CAD build for the part. Positions are in the model's coordinates, mm. Face numbers are marked on the shaded views. A direction names the side the tool comes from. Round coordinates to 2 decimals unless told otherwise and drop trailing zeros. Loops run counter-clockwise (first coordinate to the right, second up) from the corner with the lowest first, then second, coordinate; pieces in that order, holes last.
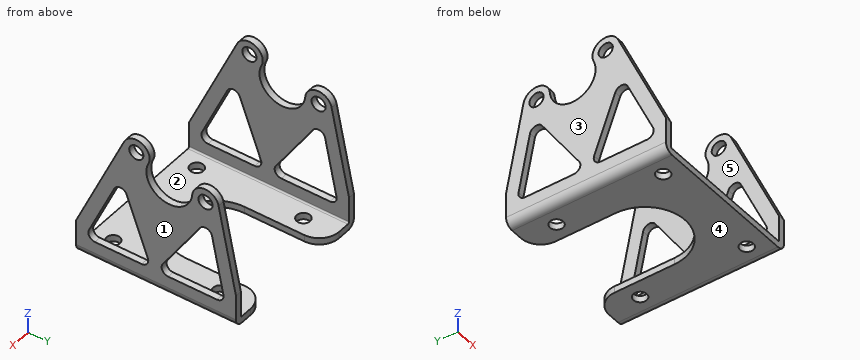
```python
from build123d import *

# Parameters (mm, degrees)
SKETCH4_R                      = 3.175
BASE_FLANGE1_DEPTH             = 3.175
EDGE_FLANGE1_STRIP_W           = 14.1732
EDGE_FLANGE1_STRIP_H           = 3.175
EDGE_FLANGE1_STRIP_CUT_DEPTH   = 76.2
EDGE_FLANGE1_STRIP_2_W         = 14.1732
EDGE_FLANGE1_STRIP_2_H         = 3.175
EDGE_FLANGE1_STRIP_CUT_2_DEPTH = 76.2
EDGE_FLANGE1_DEPTH             = 76.2
EDGE_FLANGE1_BEND_DEPTH        = 76.2
CUT_EXTRUDE2_DEPTH             = 113.499830191
CUT_EXTRUDE3_REACH             = 110.728
SKETCH21_R                     = 3.3782


# Sheet-metal steps are written as plain solids
with BuildPart() as part:
    # Sketch4 → Base-Flange1 (new body)
    with BuildSketch(Plane.XY):
        with BuildLine():
            Line((38.470301513, 37.249760359), (28.945301513, 37.249760359))
            ThreePointArc((28.945301513, 37.249760359), (22.210109423, 34.45995245), (19.420301513, 27.724760359))
            Line((19.420301513, 27.724760359), (19.420301513, -0.850239641))
            ThreePointArc((19.420301513, -0.850239641), (0.370301513, -19.900239641), (-18.679698487, -0.850239641))
            Line((-18.679698487, -0.850239641), (-18.679698487, 27.724760359))
            ThreePointArc((-18.679698487, 27.724760359), (-21.469506396, 34.45995245), (-28.204698487, 37.249760359))
            Line((-28.204698487, 37.249760359), (-37.729698487, 37.249760359))
            Line((-37.729698487, 37.249760359), (-37.729698487, -38.950239641))
            Line((-37.729698487, -38.950239641), (38.470301513, -38.950239641))
            Line((38.470301513, -38.950239641), (38.470301513, 37.249760359))
        make_face()
        with Locations((-26.617198487, -29.425239641)):
            Circle(SKETCH4_R, mode=Mode.SUBTRACT)
        with Locations((27.357801513, -29.425239641)):
            Circle(SKETCH4_R, mode=Mode.SUBTRACT)
        with Locations((27.357801513, 21.374760359)):
            Circle(SKETCH4_R, mode=Mode.SUBTRACT)
        with Locations((-26.617198487, 21.374760359)):
            Circle(SKETCH4_R, mode=Mode.SUBTRACT)
    extrude(amount=-BASE_FLANGE1_DEPTH)

    # Edge-Flange1 strip (across the edge) → Edge-Flange1 strip cut (cut)
    with BuildSketch(Plane(origin=(38.470301513, -38.950239641, 0), x_dir=(-1, 0, 0), z_dir=(0, 1, 0))):
        with Locations((-3.175, -1.5875)):
            Rectangle(EDGE_FLANGE1_STRIP_W, EDGE_FLANGE1_STRIP_H)
    extrude(amount=EDGE_FLANGE1_STRIP_CUT_DEPTH, mode=Mode.SUBTRACT)

    # Edge-Flange1 strip 2 (across the edge) → Edge-Flange1 strip cut 2 (cut)
    with BuildSketch(Plane(origin=(-37.729698487, 37.249760359, 0), x_dir=(1, 0, 0), z_dir=(0, -1, 0))):
        with Locations((-3.175, -1.5875)):
            Rectangle(EDGE_FLANGE1_STRIP_2_W, EDGE_FLANGE1_STRIP_2_H)
    extrude(amount=EDGE_FLANGE1_STRIP_CUT_2_DEPTH, mode=Mode.SUBTRACT)

    # Edge-Flange1 section (across the edge) → Edge-Flange1 (add)
    with BuildSketch(Plane(origin=(38.470301513, -38.950239641, 0), x_dir=(-1, 0, 0), z_dir=(0, 1, 0))):
        with BuildLine():
            Line((0, 0.7366), (0, 73.025))
            Line((0, 73.025), (3.175, 73.025))
            Line((3.175, 73.025), (3.175, 0.7366))
            ThreePointArc((3.175, 0.7366), (3.390745145, 0.215745145), (3.9116, 0))
            Line((3.9116, 0), (3.9116, -3.175))
            ThreePointArc((3.9116, -3.175), (1.145681115, -2.029318885), (0, 0.7366))
        make_face()
    extrude(amount=EDGE_FLANGE1_DEPTH)

    # Edge-Flange1 section 2 (across the edge) → Edge-Flange1 bend (add)
    with BuildSketch(Plane(origin=(-37.729698487, 37.249760359, 0), x_dir=(1, 0, 0), z_dir=(0, -1, 0))):
        with BuildLine():
            Line((0, 0.7366), (0, 73.025))
            Line((0, 73.025), (3.175, 73.025))
            Line((3.175, 73.025), (3.175, 0.7366))
            ThreePointArc((3.175, 0.7366), (3.390745145, 0.215745145), (3.9116, 0))
            Line((3.9116, 0), (3.9116, -3.175))
            ThreePointArc((3.9116, -3.175), (1.145681115, -2.029318885), (0, 0.7366))
        make_face()
    extrude(amount=EDGE_FLANGE1_BEND_DEPTH)

    # Sketch18 → Cut-Extrude2 (cut, through all)
    with BuildSketch(Plane(origin=(38.470301513, 0, 0), x_dir=(0, 0, -1), z_dir=(1, 0, 0))):
        with BuildLine():
            Line((-12.7, 37.249760359), (-53.545242344, 28.944361059))
            ThreePointArc((-53.545242344, 28.944361059), (-58.617648241, 22.326829154), (-52.763048756, 16.390104891))
            ThreePointArc((-52.763048756, 16.390104891), (-43.013397441, 2.790344649), (-58.09955595, -4.449613972))
            ThreePointArc((-58.09955595, -4.449613972), (-66.503585183, -7.614624659), (-63.338574497, -16.018653892))
            Line((-63.338574497, -16.018653892), (-12.7, -38.950239641))
            Line((-12.7, -38.950239641), (-73.025, -38.950239641))
            Line((-73.025, -38.950239641), (-73.025, 37.249760359))
            Line((-73.025, 37.249760359), (-12.7, 37.249760359))
        make_face()
    extrude(amount=-CUT_EXTRUDE2_DEPTH, mode=Mode.SUBTRACT)

    # Cut-Extrude3: up to this face of the body (flat: up to its plane)
    cut_extrude3_end = Plane(part.part.faces().sort_by_distance((-37.729698487, 0.375360162, 25.894827333))[0])
    # Sketch21 → Cut-Extrude3 (cut, up to the picked face)
    with BuildSketch(Plane(origin=(38.470301513, 0, 0), x_dir=(0, 0, -1), z_dir=(1, 0, 0)), mode=Mode.PRIVATE) as cut_extrude3_sk1:
        with Locations((-60.719065223, -10.234133932)):
            Circle(SKETCH21_R)
    cut_extrude3_tool1 = split(extrude(cut_extrude3_sk1.sketch, amount=-CUT_EXTRUDE3_REACH, mode=Mode.PRIVATE), bisect_by=cut_extrude3_end, keep=Keep.BOTH, mode=Mode.PRIVATE)
    # Sketch21 → Cut-Extrude3 (cut, up to the picked face)
    with BuildSketch(Plane(origin=(38.470301513, 0, 0), x_dir=(0, 0, -1), z_dir=(1, 0, 0)), mode=Mode.PRIVATE) as cut_extrude3_sk2:
        with Locations((-52.279937568, 22.721700549)):
            Circle(SKETCH21_R)
    cut_extrude3_tool2 = split(extrude(cut_extrude3_sk2.sketch, amount=-CUT_EXTRUDE3_REACH, mode=Mode.PRIVATE), bisect_by=cut_extrude3_end, keep=Keep.BOTH, mode=Mode.PRIVATE)
    # Sketch21 → Cut-Extrude3 (cut, up to the picked face)
    with BuildSketch(Plane(origin=(38.470301513, 0, 0), x_dir=(0, 0, -1), z_dir=(1, 0, 0)), mode=Mode.PRIVATE) as cut_extrude3_sk3:
        with BuildLine():
            Line((-10.64400026, -4.738220863), (-37.435582613, -14.828100623))
            ThreePointArc((-37.435582613, -14.828100623), (-39.489903551, -17.696138128), (-37.62633699, -20.691633633))
            Line((-37.62633699, -20.691633633), (-10.834754637, -32.824152651))
            ThreePointArc((-10.834754637, -32.824152651), (-7.804221974, -32.600140782), (-6.35, -29.931892671))
            Line((-6.35, -29.931892671), (-6.35, -7.709493893))
            ThreePointArc((-6.35, -7.709493893), (-7.718373423, -5.09860795), (-10.64400026, -4.738220863))
        make_face()
    cut_extrude3_tool3 = split(extrude(cut_extrude3_sk3.sketch, amount=-CUT_EXTRUDE3_REACH, mode=Mode.PRIVATE), bisect_by=cut_extrude3_end, keep=Keep.BOTH, mode=Mode.PRIVATE)
    # Sketch21 → Cut-Extrude3 (cut, up to the picked face)
    with BuildSketch(Plane(origin=(38.470301513, 0, 0), x_dir=(0, 0, -1), z_dir=(1, 0, 0)), mode=Mode.PRIVATE) as cut_extrude3_sk4:
        with BuildLine():
            Line((-38.069272281, 20.080292762), (-11.277689928, 2.343110591))
            ThreePointArc((-11.277689928, 2.343110591), (-8.022363238, 2.193595711), (-6.35, 4.990506107))
            Line((-6.35, 4.990506107), (-6.35, 28.175441224))
            ThreePointArc((-6.35, 28.175441224), (-7.516025925, 30.634027844), (-10.157652388, 31.286771479))
            Line((-10.157652388, 31.286771479), (-36.949234742, 25.839018533))
            ThreePointArc((-36.949234742, 25.839018533), (-39.433182282, 23.333848227), (-38.069272281, 20.080292762))
        make_face()
    cut_extrude3_tool4 = split(extrude(cut_extrude3_sk4.sketch, amount=-CUT_EXTRUDE3_REACH, mode=Mode.PRIVATE), bisect_by=cut_extrude3_end, keep=Keep.BOTH, mode=Mode.PRIVATE)
    add(cut_extrude3_tool1.solids().sort_by(Axis((38.470302, -10.234134, 60.719065), (-1, 0, 0)))[0], mode=Mode.SUBTRACT)
    add(cut_extrude3_tool2.solids().sort_by(Axis((38.470302, 22.721701, 52.279938), (-1, 0, 0)))[0], mode=Mode.SUBTRACT)
    add(cut_extrude3_tool3.solids().sort_by(Axis((38.470302, -18.49522, 18.845957), (-1, 0, 0)))[0], mode=Mode.SUBTRACT)
    add(cut_extrude3_tool4.solids().sort_by(Axis((38.470302, 18.532132, 18.821153), (-1, 0, 0)))[0], mode=Mode.SUBTRACT)


solid = part.part
```
Item 1: Cut at B-B, the plane z = 21. Give the cut face in (x, y).
Answers follow:
outline: (-37.73, -35.19) - (-34.55, -35.19) - (-34.55, -28.22) - (-37.73, -28.22) - close; (-37.73, -8.64) - (-34.55, -8.64) - (-34.55, 8.78) - (-37.73, 8.78) - close; (-37.73, 29.08) - (-34.55, 29.08) - (-34.55, 35.56) - (-37.73, 35.56) - close; (35.3, -35.19) - (38.47, -35.19) - (38.47, -28.22) - (35.3, -28.22) - close; (35.3, -8.64) - (38.47, -8.64) - (38.47, 8.78) - (35.3, 8.78) - close; (35.3, 29.08) - (38.47, 29.08) - (38.47, 35.56) - (35.3, 35.56) - close
Item 2: 3-axis set-ups, long thin cutter, end or side, ignore diameter. For the marked faces 1 and 2: which of +Z, -Z, +X, -X, +Y, -Y reach the whole face in a straight line?
Answers follow:
face 1: +Z, -Z, +X, +Y, -Y
face 2: +Z, +Y, -Y
Item 3: Two-plate mould, pull along X, no slides. Class the marked faces 3, 4 and 5: released by +X, released by -X, zero draft, split by the parting line, or undercut.
Answers follow:
face 3: released by -X
face 4: zero draft
face 5: undercut
Item 4: Cut at D-D, the plane x = 27.5. Give the cut face in (y, z) (3 decimals), plus the area to 3 significant figures.
Answers follow:
outline: (-38.95, -3.175) - (-32.597, -3.175) - (-32.597, 0) - (-38.95, 0) - close; (-26.253, -3.175) - (18.203, -3.175) - (18.203, 0) - (-26.253, 0) - close; (24.547, -3.175) - (37.139, -3.175) - (37.139, 0) - (24.547, 0) - close
area: 201 mm2
Item 5: Cut at A-A, the plane z = 2. Give the cut face in (x, y).
Answers follow:
outline: (-37.73, -38.95) - (-34.55, -38.95) - (-34.55, 37.25) - (-37.73, 37.25) - close; (35.3, -38.95) - (38.47, -38.95) - (38.47, 37.25) - (35.3, 37.25) - close
Item 6: Flat gauge pins, fed straight in: P1, Ø10, axis at x = -26.62, y = 21.37, coming from the -Z side (3 decimals); P2, Ø4, axis at x = 27.36, y = 21.37, coming from the +Z side; P3, Ø3.5, axis at x = -37, y = 20, coming from the +Z side; P4, Ø3.5, axis at y = 6.5, z = -1.5, coming from the -X side. Where does each tip first touch, or does it go through?
Answers follow:
P1: stops at z = -3.175
P2: passes through
P3: stops at z = 58.56
P4: stops at x = -37.7
Item 7: Probe line 1 (X direction, y = 1, z = 28.5); line 2 (Z direction, x = 21, y = -23.5) (3 decimals). List the from-to ranges inside material, lowest first.
Answers follow:
line 1: x = -37.73 to -34.55, 35.3 to 38.47
line 2: z = -3.175 to 0
Item 8: Cut at C-C, the plane y = 6.5. Give the cut face in (x, z) (3 decimals), plus the area to 3 significant figures.
Answers follow:
outline: (-37.73, 0.737) arc R3.912 ccw to (-33.818, -3.175) - (-18.68, -3.175) - (-18.68, 0) - (-33.818, 0) arc R0.737 cw to (-34.555, 0.737) - (-34.555, 6.35) - (-37.73, 6.35) - close; (-37.73, 17.557) - (-34.555, 17.557) - (-34.555, 42.718) - (-37.73, 42.718) - close; (19.42, -3.175) - (34.559, -3.175) arc R3.912 ccw to (38.47, 0.737) - (38.47, 6.35) - (35.295, 6.35) - (35.295, 0.737) arc R0.737 cw to (34.559, 0) - (19.42, 0) - close; (35.295, 17.557) - (38.47, 17.557) - (38.47, 42.718) - (35.295, 42.718) - close
area: 315 mm2
